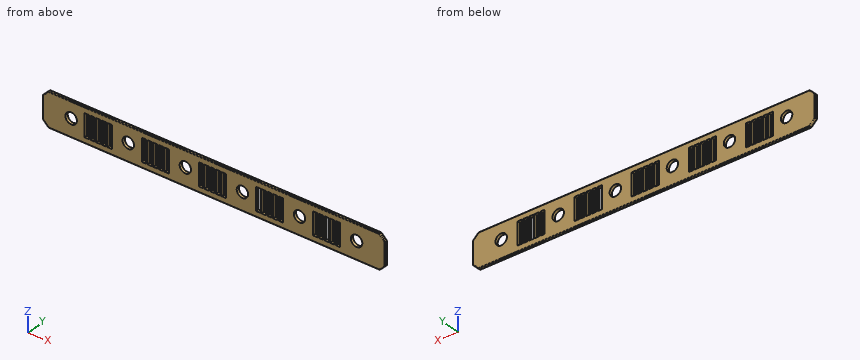
```python
from build123d import *

# Parameters (mm, degrees)
F0_W     = 762
F0_H     = 76.2
F0_R     = 12.7
F1_DEPTH = 6.35
F2_W     = 9.525
F2_H     = 50.8
F3_DEPTH = 6.351
F4_SIZE  = 12.7
F5_R     = 1.6002


with BuildPart() as f1:
    # F0 (on Front) → F1 (new body)
    with BuildSketch(Plane.XZ):
        with Locations((317.5, -2.3671598174)):
            Rectangle(F0_W, F0_H)
        Circle(F0_R, mode=Mode.SUBTRACT)
        with Locations((127, 0)):
            Circle(F0_R, mode=Mode.SUBTRACT)
        with Locations((254, 0)):
            Circle(F0_R, mode=Mode.SUBTRACT)
        with Locations((381, 0)):
            Circle(F0_R, mode=Mode.SUBTRACT)
        with Locations((508, 0)):
            Circle(F0_R, mode=Mode.SUBTRACT)
        with Locations((635, 0)):
            Circle(F0_R, mode=Mode.SUBTRACT)
    extrude(amount=F1_DEPTH)

    # F2 (on face) → F3 (cut, through all)
    with BuildSketch(Plane.XZ.offset(6.35)):
        with Locations((34.9377, -2.3671598174)):
            Rectangle(F2_W, F2_H)
        with Locations((47.6377, -2.3671598174)):
            Rectangle(F2_W, F2_H)
        with Locations((60.3377, -2.3671598174)):
            Rectangle(F2_W, F2_H)
        with Locations((73.0377, -2.3671598174)):
            Rectangle(F2_W, F2_H)
        with Locations((85.7377, -2.3671598174)):
            Rectangle(F2_W, F2_H)
        with Locations((161.9377, -2.3671598174)):
            Rectangle(F2_W, F2_H)
        with Locations((174.6377, -2.3671598174)):
            Rectangle(F2_W, F2_H)
        with Locations((187.3377, -2.3671598174)):
            Rectangle(F2_W, F2_H)
        with Locations((200.0377, -2.3671598174)):
            Rectangle(F2_W, F2_H)
        with Locations((212.7377, -2.3671598174)):
            Rectangle(F2_W, F2_H)
        with Locations((288.9377, -2.3671598174)):
            Rectangle(F2_W, F2_H)
        with Locations((301.6377, -2.3671598174)):
            Rectangle(F2_W, F2_H)
        with Locations((314.3377, -2.3671598174)):
            Rectangle(F2_W, F2_H)
        with Locations((327.0377, -2.3671598174)):
            Rectangle(F2_W, F2_H)
        with Locations((339.7377, -2.3671598174)):
            Rectangle(F2_W, F2_H)
        with Locations((415.9377, -2.3671598174)):
            Rectangle(F2_W, F2_H)
        with Locations((428.6377, -2.3671598174)):
            Rectangle(F2_W, F2_H)
        with Locations((441.3377, -2.3671598174)):
            Rectangle(F2_W, F2_H)
        with Locations((454.0377, -2.3671598174)):
            Rectangle(F2_W, F2_H)
        with Locations((466.7377, -2.3671598174)):
            Rectangle(F2_W, F2_H)
        with Locations((542.9377, -2.3671598174)):
            Rectangle(F2_W, F2_H)
        with Locations((555.6377, -2.3671598174)):
            Rectangle(F2_W, F2_H)
        with Locations((568.3377, -2.3671598174)):
            Rectangle(F2_W, F2_H)
        with Locations((581.0377, -2.3671598174)):
            Rectangle(F2_W, F2_H)
        with Locations((593.7377, -2.3671598174)):
            Rectangle(F2_W, F2_H)
    extrude(amount=-F3_DEPTH, mode=Mode.SUBTRACT)

    # F4
    f4_edges = [f1.edges().sort_by_distance(p)[0] for p in [
        (-63.5, -3.175, 35.73284),
        (-63.5, -3.175, -40.46716),
        (698.5, -3.175, 35.73284),
        (698.5, -3.175, -40.46716),
    ]]
    chamfer(f4_edges, length=F4_SIZE)

    # F5
    f5_edges = [f1.edges().sort_by_distance(p)[0] for p in [
        (317.5, -6.35, 35.73284),
        (317.5, 0, 35.73284),
        (317.5, -6.35, -40.46716),
        (317.5, 0, -40.46716),
        (-63.5, -6.35, -2.36716),
        (-63.5, 0, -2.36716),
        (698.5, -6.35, -2.36716),
        (698.5, 0, -2.36716),
        (-57.15, -6.35, -34.11716),
        (-57.15, 0, -34.11716),
        (692.15, -6.35, 29.38284),
        (692.15, 0, 29.38284),
        (692.15, -6.35, -34.11716),
        (692.15, 0, -34.11716),
        (-57.15, -6.35, 29.38284),
        (-57.15, 0, 29.38284),
    ]]
    fillet(f5_edges, radius=F5_R)


solid = f1.part
```
The model under review builds one solid part; all positions refer to its coordinate system, in mm. Coordinates: 2 decimals unless noted, no trailing zeros. Order: outer loops, then holes, each group sorted by start corner. A loop starts at its lowest first (then second) coordinate and runs counter-clockwise, first axis right, second up. Notation, with made-up numbers: (62.5, 17) -> (95.5, 17) arc R24 cw to (95.5, 29) -> close; hole circle Ø1 at (89, -21). An arc over 180 degrees is marked (long way). Answer in a Markdown table with one row per item. Add a question column.
Item 1: We need section A-A on x = 381. Write out the cut boundary in (y, z), plus the area to 3 significant figures.
Item 2: To check wall thickness, follow probe 1 along Z at (x, y) = (254, -4.5); probe 2 along Z at (x, y) = (508, -5); probe 3 along X at (y, z) = (-0.5, 31). State the ranges of each line that lie inside material, in increasing order.
Item 3: We need section B-B on z = 0. Give the number of separate pieces and of enclosed holes in the cut face, plus the area to 3 significant figures.
Final values:
| question | item | result |
|---|---|---|
| 1 | outline | (-6.35, -38.87) arc R1.6 ccw to (-4.75, -40.47) -> (-1.6, -40.47) arc R1.6 ccw to (0, -38.87) -> (0, -12.7) -> (-6.35, -12.7) -> close; (-6.35, 12.7) -> (0, 12.7) -> (0, 34.13) arc R1.6 ccw to (-1.6, 35.73) -> (-4.75, 35.73) arc R1.6 ccw to (-6.35, 34.13) -> close |
| 1 | area | 320 mm2 |
| 2 | probe 1 | z = -40.47 to -12.7, 12.7 to 35.73 |
| 2 | probe 2 | z = -40.45 to -12.7, 12.7 to 35.71 |
| 2 | probe 3 | x = -54.91 to 689.91 |
| 3 | separate pieces | 32 |
| 3 | enclosed holes | 0 |
| 3 | area | 2,360 mm2 |
